Autodesk Inventor part; units mm, degrees
ref_plane "YZ Plane" through (0, 0, 0) normal (1, 0, 0) x (0, 1, 0)
ref_plane "XZ Plane" through (0, 0, 0) normal (0, 1, 0) x (-1, 0, 0)
ref_plane "XY Plane" through (0, 0, 0) normal (0, 0, 1) x (1, 0, 0)
sketch "Sketch1" plane through (0, 0, 0) normal (0, 1, 0) x (-1, 0, 0)
  line L0 (0, 0) -> (-111.76, 0)
  line L1 (-111.76, 0) -> (-111.76, 213.36)
  line L2 (-111.76, 213.36) -> (0, 213.36)
  line L3 (0, 213.36) -> (0, 0)
  line L4 (-111.76, 212.09) -> (-111.76, 0)
  line L5 (0, 212.09) -> (-111.76, 212.09)
  line L6 (0, 0) -> (0, 212.09)
  line L7 (-111.76, 0) -> (0, 0)
  line L8 (-111.76, 0) -> (0, 0)
  line L9 (0, 0) -> (0, 212.09)
  line L10 (-111.76, 212.09) -> (-111.76, 0)
  line L11 (-111.76, 0) -> (0, 0)
  line L12 (0, 218.44) -> (-107.95, 218.44)
  line L13 (-107.95, 218.44) -> (-107.95, 212.09)
  line L14 (0, 212.09) -> (0, 218.44)
  dimension "d0" = 111.76
  dimension "d1" = 213.36
extrude "Extrusion1" add sketch "Sketch1" along normal blind 4.826 contours L0 L1 L5 L3 | L5 L13 L2 L3 | L1 L2 L13 L5
sketch "Sketch2" plane through (0, 4.826, 0) normal (0, 1, 0) x (1, 0, 0)
  line L0 (111.76, 0) -> (0, 0)
  line L1 (0, 0) -> (0, -213.36)
  line L2 (88.8491, -51.3544) -> (82.4991, -51.3544)
  line L3 (82.4991, -51.3544) -> (82.4991, -0.0669)
  line L4 (82.4991, -0.0669) -> (82.4991, -12.7669)
  line L5 (82.4991, -0.0669) -> (82.4991, -25.4669)
  circle A0 centre (82.4991, -25.4669) radius 11
  line L6 (82.4991, -25.4669) -> (82.4991, -51.8669)
  line L7 (82.4991, -36.4669) -> (82.4991, -61.8669)
  circle A1 centre (82.4928, -55.6695) radius 8.25
  line L8 (82.4991, -48.0194) -> (82.4991, -56.1194)
  line L9 (82.4928, -63.9195) -> (82.4928, -84.7195)
  circle A2 centre (82.4928, -84.7195) radius 8.25
  line L10 (82.4928, -92.9695) -> (82.4928, -113.7721)
  circle A3 centre (82.4928, -113.7721) radius 8.25
  circle A4 centre (36.0751, -176.7145) radius 11.5
  line L11 (10.6751, -176.7232) -> (36.0751, -176.7232)
  line L12 (57.6456, -16.3037) -> (16.6456, -16.3037)
  line L13 (16.6456, -16.3037) -> (16.6456, -116.3037)
  line L14 (16.6456, -116.3037) -> (57.6456, -116.3037)
  line L15 (57.6456, -116.3037) -> (57.6456, -16.3037)
  line L16 (36.0751, -176.7232) -> (36.0751, -151.3232)
  line L17 (82.8401, -122.0148) -> (82.8401, -137.2548)
  circle A5 centre (82.8401, -137.2548) radius 3.25
  line L18 (0, -213.36) -> (111.76, -213.36)
  line L19 (111.76, -213.36) -> (111.76, 0)
  dimension "d14" = 22
  dimension "d18" = 16.5
  dimension "d13" = 25.4
  dimension "d17" = 25.4
  dimension "d19" = 8.1
  dimension "d20" = 20.8
  dimension "d22" = 20.8026
  dimension "d24" = 23
  dimension "d27" = 25.4
  dimension "d28" = 41
  dimension "d29" = 100
  dimension "d30" = 25.4
  dimension "d31" = 15.24
  dimension "d32" = 6.5
extrude "Extrusion3" cut sketch "Sketch2" against normal blind 25.4 contours A0 L3 | A5 | A3 | A2 | A1 | L3 A0 | A4 L11 L16 | L16 L11 A4 | L15 L14 L13 L12
sketch "Sketch3" plane through (0, 4.826, 0) normal (0, 1, 0) x (1, 0, 0)
  circle A0 centre (82.4991, -25.4669) radius 11
  circle A1 centre (82.4928, -113.7721) radius 8.25
  line L0 (57.6456, -116.3037) -> (16.6456, -116.3037)
  line L1 (16.6456, -116.3037) -> (16.6456, -16.3037)
  line L2 (16.6456, -16.3037) -> (57.6456, -16.3037)
  line L3 (57.6456, -16.3037) -> (57.6456, -116.3037)
  circle A2 centre (82.4928, -55.6695) radius 8.25
  circle A3 centre (82.4928, -84.7195) radius 8.25
  line L4 (111.76, 0) -> (0, 0)
  line L5 (0, 0) -> (0, -213.36)
  circle A4 centre (36.0751, -176.7145) radius 11.5
  line L6 (57.6456, -116.3037) -> (16.6456, -116.3037)
  line L7 (16.6456, -116.3037) -> (16.6456, -16.3037)
  line L8 (16.6456, -16.3037) -> (57.6456, -16.3037)
  circle A5 centre (82.8401, -137.2548) radius 3.25
  line L9 (111.76, 0) -> (0, 0)
  line L10 (0, 0) -> (0, -213.36)
  line L11 (0, 0) -> (0, -213.36)
  circle A6 centre (36.0751, -176.7145) radius 11.5
  circle A7 centre (82.8401, -137.2548) radius 3.25
  line L12 (57.6456, -16.3037) -> (57.6456, -116.3037)
  line L13 (0, -213.36) -> (111.76, -213.36)
  line L14 (111.76, -213.36) -> (111.76, 0)
  point P0 (107.95, -122.8721)
  point P1 (107.95, -24.8721)
  point P2 (107.95, 0)
sketch "Sketch5" plane through (0, 4.826, 0) normal (0, 1, 0) x (1, 0, 0)
  line L0 (0, 0) -> (0, -213.36)
  line L1 (0, -213.36) -> (0, -208.36)
  circle A0 centre (8.81, -8.81) radius 2
  circle A1 centre (8.81, -207.09) radius 2
  circle A2 centre (105.49, -207.09) radius 2
  circle A3 centre (105.49, -8.81) radius 2
  circle A4 centre (105.49, -8.81) radius 2
  circle A5 centre (105.49, -207.09) radius 2
  circle A6 centre (8.81, -207.09) radius 2
  circle A7 centre (8.81, -8.81) radius 2
  dimension "d36" = 5
extrude "Extrusion5" cut sketch "Sketch5" against normal up to next
properties part number "component box cover"
Could you check a few things on this model? Use its own coordinates, in mm. A direction names the side the tool comes from. Give positions to 0.01 mm unless a question says otherwise; leave off trailing zeros. Write each loop counter-clockwise with the first axis right and the second up, starting at its lowest first coordinate (ties: lowest second). Pieces come first, ordered by that corner, then holes. Notation, with made-up numbers: (-40, -8.5) - (-6, -8.5) arc R27 cw to (-6, 19.5) - close; hole circle Ø3 at (64, 33.5). An arc over 180 degrees is marked (long way). One line per item, written item: value. Start each with the question number.
Item 1: Imagine slicing it at C-C, the plane y = 0.85. Give the number of separate pieces and of enclosed holes in the cut face, and give its area (3 significant figures).
Item 2: Imagine slicing it at A-A, the plane z = 8.81. List the corners of the cut face in (x, y) for me, and give its area (3 significant figures).
Item 3: Which directions (+Z, -Z, +X, -X, +Y, -Y) give clear straight access to the entire face, cutting with the end or side of a thin tool? Please do faces 1 (the face through (37, 2, 16.304)), 2 (the face through (69, 4.826, 108)).
Item 4: I'm going to push flat-ended pins straight in: pin 1 (3 mm diameter, centred on x = 8.81, z = 8.81, fed in from +Y); pin 2 (1 mm diameter, centred on y = 1, z = 172.5, fed in from -X). Where does each tip first touch, or does it pass through?
Item 5: If we mould it in two halves opening along Z, with no side actions, what happens to faces 3 (the face through (16.646, 2, 66)), 4 (the face through (111.76, 2, 105)), 5 (the face through (55, 2, 0))? For each: +Z half, -Z half, draft (parallel to the pull), parting line (faces both ways), or undercut.
Item 6: Please list where these lines run through material, in increasing order: line 1 (X direction, y = 0.2, z = 114); line 2 (X direction, y = 2.3, z = 9); line 3 (Z direction, x = 90, y = 1.05). Write a range as from..to.
Item 7: Imagine slicing it at B-B, the plane x = 8.81. List the corners of the cut face in (y, z) for me.
Geometry says:
1. separate pieces: 1
1. enclosed holes: 11
1. area: 18,200 mm^2
2. outline: (0, 0) - (6.81, 0) - (6.81, 4.83) - (0, 4.83) - close; (10.81, 0) - (103.49, 0) - (103.49, 4.83) - (10.81, 4.83) - close; (107.49, 0) - (111.76, 0) - (111.76, 4.83) - (107.49, 4.83) - close
2. area: 501 mm^2
3. face 1: +Y, -Y
3. face 2: +Z, -Z, +X, -X, +Y
4. pin 1: through
4. pin 2: x = 0
5. face 3: undercut
5. face 4: draft
5. face 5: -Z half
6. line 1: 0..16.65, 57.65..74.25, 90.74..111.76
6. line 2: 0..6.82, 10.8..103.5, 107.48..111.76
6. line 3: 0..17.42, 33.51..52.25, 59.09..81.3, 88.14..110.35, 117.19..213.36
7. outline: (0, 0) - (4.83, 0) - (4.83, 6.81) - (0, 6.81) - close; (0, 10.81) - (4.83, 10.81) - (4.83, 205.09) - (0, 205.09) - close; (0, 209.09) - (4.83, 209.09) - (4.83, 213.36) - (0, 213.36) - close
